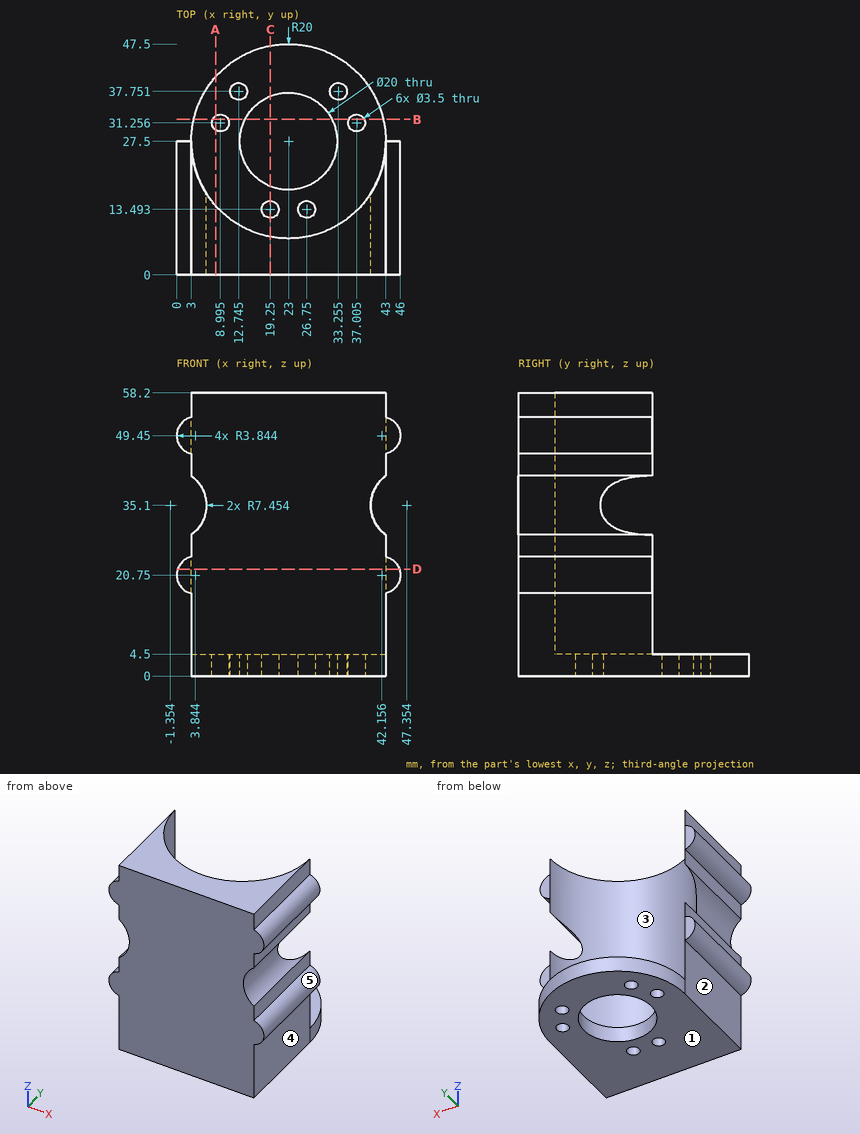
Geometry check sheet. Reference: drawing and pictorial views, mm from the part's lowest x, y, z. A direction names the side the tool comes from. Give positions to 0.01 mm unless a question says otherwise; leave off trailing zeros. Write each loop counter-clockwise with the first axis right and the second up, starting at its lowest first coordinate (ties: lowest second). Pieces come first, ordered by that corner, then holes. Notation, with made-up numbers: M -6,-15 L 42,-15 A27 cw 42,15 Z; hole C 86.25,54.25 d1. An arc over 180 degrees is marked long. Answer as CSV lines item,"result". Start each with the question number.
Q1. Section check B-B, the plane y = 32. Record the cut outline in (x, z).
Q2. Section check C-C, the plane x = 19.25. Record the cut outline in (y, z) (1 decimal).
Q3. Section check A-A, the plane x = 8. Record the cut outline in (y, z) (1 decimal).
Q4. Tool access check on the marked faces 1, 2, 3, 4 and 5. Record the directions out of +Z, -Z, +X, -X, +Y, -Y that give a thin tool (end or side, any length) a straight path to the whole face; none if there is none.
Q5. Material ranges on L1, parallel to X at y = 27, z = 2; L2, parallel to Z at x = 41, y = 32.5; L3, parallel to X at y = 13.5, z = 41.5 (1 decimal), recorded low to high.
Q6. Go/stop test with flat-tipped pins: pin 1 (5.5 mm diameter, centred on x = 26.75, y = 13.49, fed in from +Z); pin 2 (2.5 mm diameter, centred on y = 19.5, z = 44, fed in from -X); pin 3 (1.4 mm diameter, centred on y = 16, z = 27, fed in from +X); pin 4 (3 mm diameter, centred on x = 37.01, y = 31.26, fed in from +Z). Record where each tip stops, or that it passes through.
Q7. Section check D-D, the plane z = 22. Record the cut outline in (x, y).
Geometry says:
1,outline,"M 3.51,0 L 7.41,0 L 7.41,4.5 L 3.51,4.5 Z; M 10.58,0 L 14.07,0 L 14.07,4.5 L 10.58,4.5 Z; M 31.93,0 L 35.42,0 L 35.42,4.5 L 31.93,4.5 Z; M 38.59,0 L 42.49,0 L 42.49,4.5 L 38.59,4.5 Z"
2,outline,"M 0,0 L 11.7,0 L 11.7,4.5 L 7.9,4.5 L 7.9,58.2 L 0,58.2 Z; M 15.2,0 L 18.2,0 L 18.2,4.5 L 15.2,4.5 Z; M 36.8,0 L 47.1,0 L 47.1,4.5 L 36.8,4.5 Z"
3,outline,"M 0,0 L 29.8,0 L 29.8,4.5 L 14.3,4.5 L 14.3,58.2 L 0,58.2 Z; M 32.7,0 L 40.7,0 L 40.7,4.5 L 32.7,4.5 Z"
4,face 1,"-Z, +X, -X, +Y, -Y"
4,face 2,"-Z, -X, +Y, -Y"
4,face 3,"+Z, +Y"
4,face 4,"-Z, +X, +Y, -Y"
4,face 5,"+X, +Y, -Y"
5,L1,"3 to 13.01, 32.99 to 43"
5,L2,"0 to 4.5"
5,L3,"3 to 8.7, 37.3 to 43"
6,pin 1,"z = 4.5"
6,pin 2,"x = 3"
6,pin 3,"x = 43"
6,pin 4,"through"
7,outline,"M 0.21,0 L 45.79,0 L 45.79,27.5 L 43,27.5 A20 cw 3,27.5 L 0.21,27.5 Z"
